The listing builds one solid part. Answer for the finished solid, in the listing's coordinates (mm). A direction names the side the tool comes from. Coordinates: 2 decimals unless noted, no trailing zeros. Loops run counter-clockwise (first coordinate to the right, second up) from the corner with the lowest first, then second, coordinate; pieces in that order, holes last. Notation, with made-up numbers: (54, 3.5) - (86, 3.5) arc R26 cw to (86, 17.5) - close; hole circle Ø10 at (61.5, 29.25). An arc over 180 degrees is marked (long way). Put each result on its own line as item: value.
```python
from build123d import *

# Parameters (mm, degrees)
SKETCH_1_R      = 2
EXTRUDE_1_DEPTH = 5


with BuildPart() as part:
    # 草图1 → 凸台-拉伸1 (new body)
    with BuildSketch(Plane(origin=(0, 0, 0), x_dir=(0, 0, -1), z_dir=(1, 0, 0))):
        Polygon((0, 0), (-250, 0), (-250, 20), (-245, 20), (-245, 70), (-250, 70), (-250, 90), (0, 90), (0, 70), (-5, 70), (-5, 20), (0, 20), align=None)
        with Locations((-40, 70)):
            Circle(SKETCH_1_R, mode=Mode.SUBTRACT)
        with Locations((-40, 20)):
            Circle(SKETCH_1_R, mode=Mode.SUBTRACT)
        with Locations((-187.5, 20)):
            Circle(SKETCH_1_R, mode=Mode.SUBTRACT)
        with Locations((-190, 70)):
            Circle(SKETCH_1_R, mode=Mode.SUBTRACT)
    extrude(amount=EXTRUDE_1_DEPTH)


solid = part.part
```
1) The part is cut by section A-A (x = 0.9). Give the vertices of the cut face in (y, z), and give its area (3 significant figures).
Found:
outline: (0, 0) - (20, 0) - (20, 5) - (70, 5) - (70, 0) - (90, 0) - (90, 250) - (70, 250) - (70, 245) - (20, 245) - (20, 250) - (0, 250) - close; hole circle Ø4 at (20, 40); hole circle Ø4 at (20, 187.5); hole circle Ø4 at (70, 40); hole circle Ø4 at (70, 190)
area: 21,900 mm^2
2) For a pull along Y with two mould halves and no side action, classify faces 1 (the face through (2, 10, 0)), 2 (the face through (2, 70, 247)), 3 (the face through (2, 0, 123)), 4 (the face through (2, 90, 127)) as pulls with the +Y half, pulls with the -Y half, needs draft (parallel to the pull), parting line crosses it, or undercut.
Found:
face 1: needs draft
face 2: undercut
face 3: pulls with the -Y half
face 4: pulls with the +Y half
3) Each of these flat-tipped pins is pushed along its axis until it touches: pin 1 (2.5 mm diameter, centred on y = 70, z = 40, fed in from -X); pin 2 (1.5 mm diameter, centred on x = 2.5, y = 39.5, fed in from -Z); pin 3 (1.5 mm diameter, centred on x = 2, y = 41, fed in from +Z). Where does it stop, or does it pass through?
Found:
pin 1: passes through
pin 2: stops at z = 5
pin 3: stops at z = 245
4) Straight lines are drawn through the part: L1, parallel to Y at x = 2.8, z = 40; L2, parallel to Y at x = 3.55, z = 187.5; L3, parallel to Z at x = 2.2, y = 34.5. For each, find the intervals that lie inside material, in ascending order. Write a range as [from, to].
Found:
L1: y = [0, 18], [22, 68], [72, 90]
L2: y = [0, 18], [22, 90]
L3: z = [5, 245]
5) The part is cut by section B-B (y = 35). Give the vertices of the cut face in (x, z), and give its area (3 significant figures).
Found:
outline: (0, 5) - (5, 5) - (5, 245) - (0, 245) - close
area: 1,200 mm^2
6) For faces 5 (the face through (2, 70, 2)), 6 (the face through (2, 20, 248)), 7 (the face through (2.465, 71.352, 191.474)), determine the directions among +Z, -Z, +X, -X, +Y, -Y from which every point of the face is accessible in a straight line to the end or side of a thin tool.
Found:
face 5: -Z, +X, -X
face 6: +Z, +X, -X
face 7: +X, -X
